Source: CAD feature listing. Evaluate the final solid. Frame: model axes, mm. Round coordinates to 2 decimals unless told otherwise and drop trailing zeros. Order: outer loops, then holes, each group sorted by start corner. A loop starts at its lowest first (then second) coordinate and runs counter-clockwise, first axis right, second up. Notation, with made-up numbers: (-37.5, 40) - (5.5, 40) arc R37 ccw to (5.5, 78) - close; hole circle Ø8 at (-38.5, 89.5). An arc over 180 degrees is marked (long way). Put each result on its own line as item: value. Start each with the question number.
1) Section A-A on x = 0. Output: boundary loops of the cut face in (y, z), then the cut area to 3 significant figures.
2) Section C-C on y = -33. Output: boundary loops of the cut face in (x, z).
3) Section B-B on z = 576. Output: boundary loops of the cut face in (x, y), then the cut area to 3 significant figures.
4) Line query: probe 1 along Z at (x, y) = (0, -27.5); probe 2 along X at (y, z) = (-55.5, 0); probe 3 along Z at (x, y) = (-779.5, -78.5). Output: solid intervals per line, ascending. Write a range as [from, to].
5) Contact query for flat-ended pins moving along their axis: P1, Ø8, axis at x = 133, y = -84.5, coming from the -Z side; P2, Ø8, axis at x = 198, y = -38, coming from the +Z side; P3, Ø6, axis at x = 388.5, y = -40, coming from the +Z side. Output: stop coordinate, or through.
6) Section D-D on z = 0. Output: boundary loops of the cut face in (x, y).
```python
from build123d import *

# Parameters (mm, degrees)
F1_DEPTH = 100
F4_W     = 100
F4_H     = 500
F5_DEPTH = 100
F7_DEPTH = 100


with BuildPart() as f1:
    # F0 (on Front) → F1 (new body)
    with BuildSketch(Plane.XZ):
        with BuildLine():
            ThreePointArc((-707.1067811865, 250), (126.8264840443, 739.1989197401), (750, 0))
            ThreePointArc((750, 0), (126.8264840443, -739.1989197401), (-707.1067811865, -250))
            Line((-707.1067811865, -250), (-968.2458365519, -250))
            ThreePointArc((-968.2458365519, -250), (126.0042924827, -992.0296962672), (1000, 0))
            ThreePointArc((1000, 0), (126.0042924827, 992.0296962672), (-968.2458365519, 250))
            Line((-968.2458365519, 250), (-707.1067811865, 250))
        make_face()
    extrude(amount=F1_DEPTH)

    # F4 (on offset) → F5 (join)
    with BuildSketch(Plane.YZ.offset(-1000)):
        with Locations((-50, -500)):
            Rectangle(F4_W, F4_H)
    extrude(amount=F5_DEPTH)

    # F6 (on face) → F7 (cut)
    with BuildSketch(Plane.XZ.offset(100)):
        with BuildLine():
            Line((-707.1067811865, -250), (-899.4680664961, -250))
            Line((-899.4680664961, -250), (-491.3664999003, -566.6206515613))
            ThreePointArc((-491.3664999003, -566.6206515613), (-619.7957007099, -422.3189427216), (-707.1067811865, -250))
        make_face()
    extrude(amount=-F7_DEPTH, mode=Mode.SUBTRACT)


solid = f1.part
```
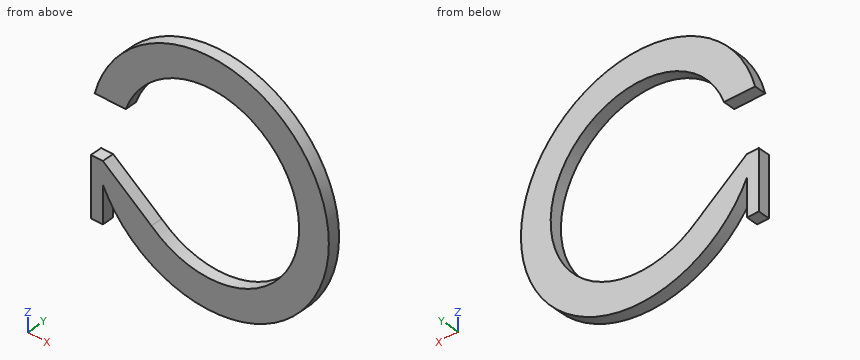
Answer sheet:
1. outline: (-100, -1000) - (0, -1000) - (0, -750) - (-100, -750) - close; (-100, 750) - (0, 750) - (0, 1000) - (-100, 1000) - close
1. area: 50,000 mm^2
2. outline: (-1000, -750) - (-900, -750) - (-900, -435.89) arc R1000 ccw (long way) to (-968.25, 250) - (-707.11, 250) arc R750 cw (long way) to (-491.37, -566.62) - (-899.47, -250) - (-1000, -250) - close
3. outline: (-817.45, -100) - (-480.34, -100) - (-480.34, 0) - (-817.45, 0) - close; (480.34, -100) - (817.45, -100) - (817.45, 0) - (480.34, 0) - close
3. area: 67,400 mm^2
4. probe 1: [-1000, -750], [750, 1000]
4. probe 2: [750, 1000]
4. probe 3: [-626.4, -343.08], [250, 626.4]
5. P1: z = -991.64
5. P2: z = 981
5. P3: z = 922.71
6. outline: (750, -100) - (1000, -100) - (1000, 0) - (750, 0) - close
